from build123d import *

# Parameters (mm, degrees)
SKETCH1_R           = 4.75
SKETCH1_R_2         = 4
BOSS_EXTRUDE1_DEPTH = 10
CUT_EXTRUDE2_DEPTH  = 10
SKETCH4_W           = 8.174166442
SKETCH4_H           = 1.582309943
BOSS_EXTRUDE2_DEPTH = 1.5


with BuildPart() as part:
    # Sketch1 → Boss-Extrude1 (new body)
    with BuildSketch(Plane.XY):
        Circle(SKETCH1_R)
        Circle(SKETCH1_R_2, mode=Mode.SUBTRACT)
    extrude(amount=BOSS_EXTRUDE1_DEPTH)

    # Sketch3 → Cut-Extrude2 (cut)
    with BuildSketch(Plane.XY.offset(10)):
        with BuildLine():
            ThreePointArc((1.66450103, 3.637229209), (3.365858295, 2.161249162), (4, 0))
            Line((4, 0), (4.75, 0))
            ThreePointArc((4.75, 0), (4.749994219, 0.007410728), (4.749976876, 0.014821438))
            ThreePointArc((4.749976876, 0.014821438), (3.992947753, 2.572716122), (1.976594973, 4.319209686))
            Line((1.976594973, 4.319209686), (1.66450103, 3.637229209))
        make_face()
        with BuildLine():
            Line((4.75, 0), (4, 0))
            ThreePointArc((4, 0), (3.365858295, -2.161249162), (1.66450103, -3.637229209))
            Line((1.66450103, -3.637229209), (1.976594973, -4.319209686))
            ThreePointArc((1.976594973, -4.319209686), (3.996956725, -2.56648338), (4.75, 0))
        make_face()
    extrude(amount=-CUT_EXTRUDE2_DEPTH, mode=Mode.SUBTRACT)

    # Sketch4 → Boss-Extrude2 (add)
    with BuildSketch(Plane(origin=(-4.5, 0, 0), x_dir=(0, 0, -1), z_dir=(1, 0, 0))):
        with Locations((-5.116351143, 0.000178202)):
            Rectangle(SKETCH4_W, SKETCH4_H)
    extrude(amount=-BOSS_EXTRUDE2_DEPTH)


solid = part.part
Here's how the part is built. I have some questions about the finished solid (model axes, mm). A direction names the side the tool comes from. Coordinates: 2 decimals unless noted, no trailing zeros. Write each loop counter-clockwise with the first axis right and the second up, starting at its lowest first coordinate (ties: lowest second). Pieces come first, ordered by that corner, then holes.
1) If we section it at C-C (z = 7.75): List the corners of the cut face in (x, y) for me, plus the area to 3 significant figures.
Filled in:
outline: (-6, -0.79) - (-4.68, -0.79) arc R4.75 ccw to (1.98, -4.32) - (1.66, -3.64) arc R4 cw (long way) to (1.66, 3.64) - (1.98, 4.32) arc R4.75 ccw to (-4.68, 0.79) - (-6, 0.79) - close
area: 15.1 mm2
2) If we section it at A-A (x = 0): List the corners of the cut face in (y, z) for me, plus the area to 3 significant figures.
Filled in:
outline: (-4.75, 0) - (-4, 0) - (-4, 10) - (-4.75, 10) - close; (4, 0) - (4.75, 0) - (4.75, 10) - (4, 10) - close
area: 15.0 mm2
3) If I drill on line 1 (Y direction, x = 0, z = 6); line 2 (X direction, y = 0, z = 3.5); line 3 (Y direction, x = -1.5, z = 8.5), over which ranges is the centre line in solid material (lowest first)?
Filled in:
line 1: y = -4.75 to -4, 4 to 4.75
line 2: x = -6 to -4
line 3: y = -4.51 to -3.71, 3.71 to 4.51
4) Thinking about a two-plate mould opening in Y: for faces 3 (the face through (-4, 0, 5)), 4 (the face through (-4.14, -0.33, 0)), 5 (the face through (-5, 0.791, 5)), which applies, +Y half, -Y half, draft (parallel to the pull), parting line (faces both ways), or undercut?
Filled in:
face 3: undercut
face 4: draft
face 5: +Y half
5) If we section it at B-B (y = 0): List the corners of the cut face in (x, z) for me.
Filled in:
outline: (-6, 1.03) - (-4.75, 1.03) - (-4.75, 0) - (-4, 0) - (-4, 10) - (-4.75, 10) - (-4.75, 9.2) - (-6, 9.2) - close
6) If we section it at D-D (x = -1): List the corners of the cut face in (y, z) for me, plus the area to 3 significant figures.
Filled in:
outline: (-4.64, 0) - (-3.87, 0) - (-3.87, 10) - (-4.64, 10) - close; (3.87, 0) - (4.64, 0) - (4.64, 10) - (3.87, 10) - close
area: 15.4 mm2
7) Which directions (+Z, -Z, +X, -X, +Y, -Y) give clear straight access to the entire face, cutting with the end or side of a thin tool? Please do faces 1 (the face through (-6, 0, 5)), 2 (the face through (-5, -0.791, 5)).
Filled in:
face 1: +Z, -Z, -X, +Y, -Y
face 2: +Z, -Z, -X, -Y
8) I'm going to push flat-ended pins straight in: pin 1 (1.4 mm diameter, centred on x = -5.5, y = -0.5, fed in from -Z); pin 2 (2 mm diameter, centred on y = -1, z = 1.5, fed in from +X); pin 3 (1.4 mm diameter, centred on x = -5.5, z = 7, fed in from +Y). Where does each tip first touch, or does it pass through?
Filled in:
pin 1: stops at z = 1.03
pin 2: stops at x = -3.46
pin 3: stops at y = 0.79
